Geometry: final body of the model. Coordinates: model frame, mm. Round coordinates to 2 decimals unless told otherwise and drop trailing zeros. Loops run counter-clockwise (first coordinate to the right, second up) from the corner with the lowest first, then second, coordinate; pieces in that order, holes last. Notation, with made-up numbers: M 34.5,13 L 68.5,13 A11 cw 68.5,23 Z; hole C -39,76.25 d1. An arc over 180 degrees is marked long. Return JSON: item names as keys, results as strings.
from build123d import *

# Parameters (mm, degrees)
EXTRUDE_1_DEPTH = 350


with BuildPart() as part:
    # Model → 凸台-拉伸1 (new body)
    with BuildSketch(Plane.XY):
        with BuildLine():
            Line((1340.138554246, 805.862554257), (1345.138554246, 805.862554257))
            Line((1345.138554246, 805.862554257), (1345.138554246, 804.862554257))
            Line((1345.138554246, 804.862554257), (1342.638554246, 804.862554257))
            Line((1342.638554246, 804.862554257), (1342.638554246, 802.862554257))
            Line((1342.638554246, 802.862554257), (1355.138554246, 802.862554257))
            Line((1355.138554246, 802.862554257), (1355.138554246, 799.862554257))
            Line((1355.138554246, 799.862554257), (1344.038554246, 799.862554257))
            Line((1344.038554246, 799.862554257), (1344.038554246, 799.362554257))
            ThreePointArc((1344.038554246, 799.362554257), (1343.638554246, 798.962554257), (1343.238554246, 799.362554257))
            ThreePointArc((1343.238554246, 799.362554257), (1340.507183396, 800.493925107), (1341.638554246, 797.762554257))
            ThreePointArc((1341.638554246, 797.762554257), (1342.09519806, 797.220410998), (1341.483330886, 796.862554257))
            Line((1341.483330886, 796.862554257), (1341.138554246, 796.862554257))
            Line((1341.138554246, 796.862554257), (1341.138554246, 785.862554257))
            Line((1341.138554246, 785.862554257), (1338.138554246, 785.862554257))
            Line((1338.138554246, 785.862554257), (1338.138554246, 798.362554257))
            Line((1338.138554246, 798.362554257), (1336.138554246, 798.362554257))
            Line((1336.138554246, 798.362554257), (1336.138554246, 795.862554257))
            Line((1336.138554246, 795.862554257), (1335.138554246, 795.862554257))
            Line((1335.138554246, 795.862554257), (1335.138554246, 800.862554257))
            ThreePointArc((1335.138554246, 800.862554257), (1336.60302034, 804.398088163), (1340.138554246, 805.862554257))
        make_face()
    extrude(amount=EXTRUDE_1_DEPTH)


solid = part.part
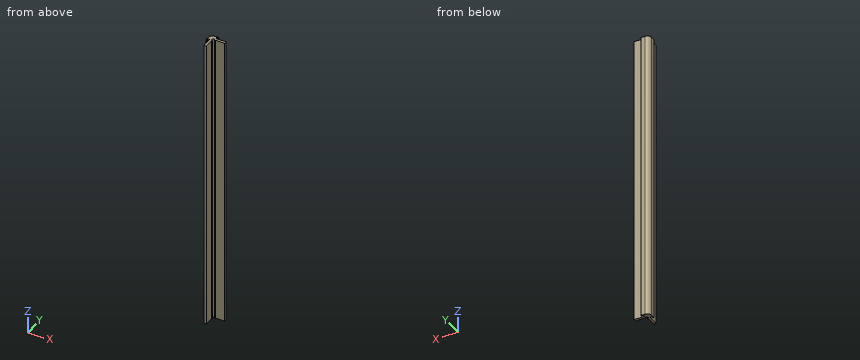
Q1. Material intervals for L1, parallel to Y at x = 1344.25, z = 253.5; L2, parallel to X at y = 799.75, z = 210.5; L3, parallel to X at y = 791.25, z = 215.5, sorted ascending.
Determined:
{"L1": "y = 799.86 to 802.86, 804.86 to 805.86", "L2": "x = 1335.14 to 1340.09, 1343.19 to 1344.04", "L3": "x = 1338.14 to 1341.14"}
Q2. Section query A-A (z = 119.5). Output: boundary loops of the cut face in (x, y), plus the area to 3 significant figures.
Determined:
{"outline": "M 1335.14,795.86 L 1336.14,795.86 L 1336.14,798.36 L 1338.14,798.36 L 1338.14,785.86 L 1341.14,785.86 L 1341.14,796.86 L 1341.48,796.86 A0.46 ccw long 1341.64,797.76 A1.6 cw long 1343.24,799.36 A0.4 ccw 1344.04,799.36 L 1344.04,799.86 L 1355.14,799.86 L 1355.14,802.86 L 1342.64,802.86 L 1342.64,804.86 L 1345.14,804.86 L 1345.14,805.86 L 1340.14,805.86 A5 ccw 1335.14,800.86 Z", "area": "126 mm^2"}
Q3. Section query B-B (y = 792.25). Output: boundary loops of the cut face in (x, z), plus the area to 3 significant figures.
Determined:
{"outline": "M 1338.14,0 L 1341.14,0 L 1341.14,350 L 1338.14,350 Z", "area": "1,050 mm^2"}
Q4. Section query C-C (x = 1349). Output: boundary loops of the cut face in (y, z), plus the area to 3 significant figures.
Determined:
{"outline": "M 799.86,0 L 802.86,0 L 802.86,350 L 799.86,350 Z", "area": "1,050 mm^2"}
Q5. Pin query (flat end, axial travel): pin 1 (4 mm diameter, centred on x = 1347.5, z = 189, fed in from +Y); pin 2 (1.5 mm diameter, centred on x = 1338, y = 792, fed in from -Z); pin 3 (1.5 mm diameter, centred on y = 791.5, z = 106.5, fed in from -X); pin 4 (5.5 mm diameter, centred on x = 1350, z = 215.5, fed in from -Y). Return the tip coordinate at first contact, or that it passes through.
Determined:
{"pin 1": "stops at y = 802.86", "pin 2": "stops at z = 0", "pin 3": "stops at x = 1338.14", "pin 4": "stops at y = 799.86"}
